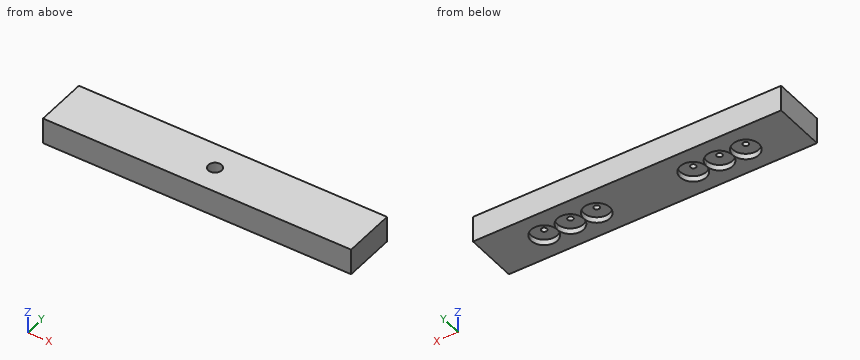
Autodesk Fusion 360 part; units mm, degrees
sketch "Boceto1" plane through (0, 0, 0) normal (0, 0, 1) x (1, 0, 0)
  line L0 (65.1, -11.1) -> (-65.1, -11.1)
  line L1 (-65.1, -11.1) -> (-65.1, 11.1)
  line L2 (-65.1, 11.1) -> (65.1, 11.1)
  line L3 (65.1, 11.1) -> (65.1, -11.1)
  line L4 (65.1, -11.1) -> (-65.1, 11.1) construction
  line L5 (-65.1, -11.1) -> (65.1, 11.1) construction
  line L6 (0, 11.1) -> (0, -11.1) construction
  line L7 (-65.1, 0) -> (65.1, 0) construction
  circle A0 centre (20.4, 0) radius 5.55
  circle A1 centre (20.4, 0) radius 1.175
  circle A2 centre (-20.4, 0) radius 5.55
  circle A3 centre (-20.4, 0) radius 1.175
  circle A4 centre (31.5, 0) radius 5.55
  circle A5 centre (31.5, 0) radius 1.175
  circle A6 centre (-31.5, 0) radius 5.55
  circle A7 centre (-31.5, 0) radius 1.175
  circle A8 centre (42.6, 0) radius 5.55
  circle A9 centre (42.6, 0) radius 1.175
  circle A10 centre (-42.6, 0) radius 1.175
  circle A11 centre (-42.6, 0) radius 5.55
  dimension "d9" = 22.2
  dimension "d14" = 11.1
  dimension "d15" = 2.35
  dimension "d16" = 20.4
  dimension "d17" = 11.1
  dimension "d18" = 2.35
  dimension "d19" = 31.5
  dimension "d20" = 11.1
  dimension "d21" = 2.35
  dimension "d22" = 42.6
  dimension "d23" = 22.5
extrude "Extruir1" add sketch "Boceto1" along normal blind 11 contours L0 L1 L2 L3 | A0 | A8 | A4 | A1 | A2 | A11 | A6 | A3 | A5 | A7 | A9 | A10
extrude "Extruir2" cut sketch "Boceto1" along normal blind 2.45 contours A0 | A8 | A4 | A2 | A11 | A6
extrude "Extruir3" cut sketch "Boceto1" along normal blind 4.9 contours A1 | A3 | A5 | A7 | A9 | A10
sketch "Boceto2" plane through (0, 0, 11) normal (0, 0, 1) x (-1, 0, 0)
  line L0 (-65.1, -11.1) -> (65.1, -11.1)
  line L1 (65.1, -11.1) -> (65.1, 11.1)
  line L2 (65.1, 11.1) -> (-65.1, 11.1)
  line L3 (-65.1, 11.1) -> (-65.1, -11.1)
  line L4 (65.1, 0) -> (-65.1, 0) construction
  line L5 (0, 11.1) -> (0, -11.1) construction
  circle A0 centre (0, 0) radius 2.8
  dimension "d31" = 5.6
extrude "Extruir4" cut sketch "Boceto2" against normal blind 6 contours A0
equation "grosor1 = 2.8 mm"
equation "grosor2 = 2 mm"
equation "grosor3 = 7.5 mm"
equation "tolerancia = 0.1 mm"
equation "diametro_grande_iman = 11 mm"
equation "diametro_pequeno_iman = 2.25 mm"
equation "altura_grande_iman = 2.45 mm"
equation "altura_pequena_iman = 2.45 mm"
equation "d9 = 18 mm + tolerancia * 2 + grosor2 * 2"
equation "DIP_pequena = 41 mm"
equation "DIP_media = 63 mm"
equation "d14 = diametro_grande_iman + tolerancia"
equation "d15 = diametro_pequeno_iman + tolerancia"
equation "d16 = ( DIP_media - ( ( diametro_grande_iman + tolerancia ) * 2 ) ) / 2"
equation "d17 = diametro_grande_iman + tolerancia"
equation "d18 = diametro_pequeno_iman + tolerancia"
equation "d19 = DIP_media / 2"
equation "d20 = diametro_grande_iman + tolerancia"
equation "d21 = diametro_pequeno_iman + tolerancia"
equation "d22 = ( DIP_media + ( ( diametro_grande_iman + tolerancia ) * 2 ) ) / 2"
equation "grosor4 = 11 mm"
equation "d27 = altura_grande_iman"
equation "d29 = altura_pequena_iman + altura_grande_iman"
equation "d31 = 5.5 mm + tolerancia"
For this review, take the finished solid that the model builds, in its own axes (mm). Give positions to 0.01 mm unless a question says otherwise; leave off trailing zeros. Order: outer loops, then holes, each group sorted by start corner. A loop starts at its lowest first (then second) coordinate and runs counter-clockwise, first axis right, second up. Notation, with made-up numbers: (-35.5, 71.25) -> (-15.5, 71.25) arc R26 cw to (-15.5, 96.25) -> close; hole circle Ø1 at (-23, 70). An arc over 180 degrees is marked (long way). Write item = value, one per line.
1) To check wall thickness, follow L1, parallel to Y at x = -20.4, z = 4.05 (3 decimals); L2, parallel to Y at x = 20.4, z = 1.2; L3, parallel to X at y = 0, z = 9.7. State the ranges of each line that lie inside material, in increasing order. Write a range as from..to.
Findings:
L1 = -11.1..-1.175, 1.175..11.1
L2 = -11.1..-5.55, 5.55..11.1
L3 = -65.1..-2.8, 2.8..65.1
2) Insertion check: pin 1 (0.7 mm diameter, centred on x = -31, y = 0, fed in from -Z); pin 2 (1.9 mm diameter, centred on x = 43, y = -0.5, fed in from -Z); pin 3 (1.7 mm diameter, centred on x = 0.5, y = 1, fed in from +Z). Each pin has a flat end and moves straight along its axis. Give the tip position at first contact, or say it passes through.
Findings:
pin_1 = 4.9
pin_2 = 2.45
pin_3 = 5
3) We need section A-A, the plane x = 42.6. Give the boundary of the cut face in (y, z) (3 decimals), and give its area (3 significant figures).
Findings:
outline = (-11.1, 0) -> (-5.55, 0) -> (-5.55, 2.45) -> (-1.175, 2.45) -> (-1.175, 4.9) -> (1.175, 4.9) -> (1.175, 2.45) -> (5.55, 2.45) -> (5.55, 0) -> (11.1, 0) -> (11.1, 11) -> (-11.1, 11) -> close
area = 211 mm^2
4) We need section B-B, the plane y = -4.25. Give the boundary of the cut face in (x, z).
Findings:
outline = (-65.1, 0) -> (-46.17, 0) -> (-46.17, 2.45) -> (-39.03, 2.45) -> (-39.03, 0) -> (-35.07, 0) -> (-35.07, 2.45) -> (-27.93, 2.45) -> (-27.93, 0) -> (-23.97, 0) -> (-23.97, 2.45) -> (-16.83, 2.45) -> (-16.83, 0) -> (16.83, 0) -> (16.83, 2.45) -> (23.97, 2.45) -> (23.97, 0) -> (27.93, 0) -> (27.93, 2.45) -> (35.07, 2.45) -> (35.07, 0) -> (39.03, 0) -> (39.03, 2.45) -> (46.17, 2.45) -> (46.17, 0) -> (65.1, 0) -> (65.1, 11) -> (-65.1, 11) -> close
5) We need section C-C, the plane x = 0. Give the boundary of the cut face in (y, z), and give its area (3 significant figures).
Findings:
outline = (-11.1, 0) -> (11.1, 0) -> (11.1, 11) -> (2.8, 11) -> (2.8, 5) -> (-2.8, 5) -> (-2.8, 11) -> (-11.1, 11) -> close
area = 211 mm^2
